```python
from build123d import *

# Parameters (mm, degrees)
SKETCH1_R           = 4.5
BOSS_EXTRUDE1_DEPTH = 5
SKETCH2_W           = 20
SKETCH2_H           = 39
BOSS_EXTRUDE2_DEPTH = 25
CUT_EXTRUDE1_DEPTH  = 30
SKETCH4_R           = 2.6
SKETCH4_R_2         = 3.2
CUT_EXTRUDE2_DEPTH  = 10
FILLET1_R           = 2
FILLET2_R           = 1


with BuildPart() as part:
    # Sketch1 → Boss-Extrude1 (new body)
    with BuildSketch(Plane.XY):
        Polygon((-10, 10), (-10, -10), (-10, -11), (10, -11), (10, -10), (10, 10), (10, 44), (-10, 44), align=None)
        with Locations((0, -0.5)):
            Circle(SKETCH1_R, mode=Mode.SUBTRACT)
    extrude(amount=BOSS_EXTRUDE1_DEPTH)

    # Sketch2 → Boss-Extrude2 (add)
    with BuildSketch(Plane(origin=(0, 0, 0), x_dir=(-1, 0, 0), z_dir=(0, 0, -1))):
        with Locations((0, 29.5)):
            Rectangle(SKETCH2_W, SKETCH2_H)
    extrude(amount=BOSS_EXTRUDE2_DEPTH)

    # Sketch3 → Cut-Extrude1 (cut)
    with BuildSketch(Plane(origin=(10, 0, 0), x_dir=(0, 0, -1), z_dir=(1, 0, 0))):
        Polygon((0, 15), (-5, 15), (-5, 49), (20, 49), (20, 15), align=None)
    extrude(amount=-CUT_EXTRUDE1_DEPTH, mode=Mode.SUBTRACT)

    # Sketch4 → Cut-Extrude2 (cut)
    with BuildSketch(Plane.XY.offset(-20)):
        with Locations((0, 40)):
            Circle(SKETCH4_R)
        with Locations((0, 25)):
            Circle(SKETCH4_R_2)
    extrude(amount=-CUT_EXTRUDE2_DEPTH, mode=Mode.SUBTRACT)

    # Fillet1
    fillet1_edges = [part.edges().sort_by_distance(p)[0] for p in [
        (0, 15, -20),
    ]]
    fillet(fillet1_edges, radius=FILLET1_R)

    # Fillet2
    fillet2_edges = [part.edges().sort_by_distance(p)[0] for p in [
        (0, 15, 5),
    ]]
    fillet(fillet2_edges, radius=FILLET2_R)


solid = part.part
```
Check sheet for the modelled part. Datum: model origin and axes. Units: mm. A direction names the side the tool comes from. Coordinates: 2 decimals unless noted, no trailing zeros. Order: outer loops, then holes, each group sorted by start corner. A loop starts at its lowest first (then second) coordinate and runs counter-clockwise, first axis right, second up. Notation, with made-up numbers: (46, 86.5) -> (89, 86.5) arc R19 ccw to (89, 102.5) -> close; hole circle Ø11 at (41, 70). An arc over 180 degrees is marked (long way). Write item = value, one per line. Start each with the question number.
1) Material ranges on L1, parallel to Y at x = 0, z = -23.4; L2, parallel to Y at x = 0, z = 1.5; L3, parallel to Y at x = -7.25, z = -14, recorded low to high.
2) Cross-section at A-A (y = -0.5). Enter the section's corners in (x, z).
3) Go/stop test with flat-tipped pins: P1, Ø3, axis at x = 3.5, z = -16.5, coming from the +Y side; P2, Ø10, axis at x = -2.5, y = -1.5, coming from the -Z side; P3, Ø6, axis at x = 1.5, z = -21, coming from the -Y side; P4, Ø8, axis at x = 0, y = -0.5, coming from the +Z side. Record where each tip stops, or that it passes through.
4) Mould release check, pull along X, two halves, no side actions. Record for faces 1 (the flat face through (-10, 14, -11)), 2 (the cylindrical face through (-0.417, 28.173, -22.465)), 3 (the flat face through (0, 33, -20)): +X half, -X half, draft (parallel to the pull), parting line (faces both ways), or undercut.
5) Cross-section at B-B (x = 0). Enter the section's corners in (y, z).
6) Access from +Z, -Z, +X, -X, +Y, -Y to the whole of each face (thin tool, end or side, straight path). Record for faces 4 (the flat face through (0, 15, -7)), 5 (the flat face through (-5, 0, 0)), 6 (the flat face through (10, 14, -11)).
7) Cross-section at C-C (z = -20.75). Enter the section's corners in (x, y), then the cut area to 3 significant figures.
8) Cross-section at D-D (y = 25). Enter the section's corners in (x, z).
Ans:
q1.L1 = 10 to 21.8, 28.2 to 37.4, 42.6 to 49
q1.L2 = -11 to -5, 4 to 15
q1.L3 = 10 to 15
q2.outline = (-10, 0) -> (-4.5, 0) -> (-4.5, 5) -> (-10, 5) -> close; (4.5, 0) -> (10, 0) -> (10, 5) -> (4.5, 5) -> close
q3.P1 = 15
q3.P2 = 0
q3.P3 = 10
q3.P4 = through
q4.face_1 = -X half
q4.face_2 = undercut
q4.face_3 = draft
q5.outline = (-11, 0) -> (-5, 0) -> (-5, 5) -> (-11, 5) -> close; (4, 0) -> (10, 0) -> (10, -25) -> (21.8, -25) -> (21.8, -20) -> (17, -20) arc R2 cw to (15, -18) -> (15, 4) arc R1 ccw to (14, 5) -> (4, 5) -> close; (28.2, -25) -> (37.4, -25) -> (37.4, -20) -> (28.2, -20) -> close; (42.6, -25) -> (49, -25) -> (49, -20) -> (42.6, -20) -> close
q6.face_4 = +Z, +X, -X, +Y
q6.face_5 = -Z, +X, -X, -Y
q6.face_6 = +Z, -Z, +X, +Y, -Y
q7.outline = (-10, 10) -> (10, 10) -> (10, 49) -> (-10, 49) -> close; hole circle Ø6.4 at (0, 25); hole circle Ø5.2 at (0, 40)
q7.area = 727 mm²
q8.outline = (-10, -25) -> (-3.2, -25) -> (-3.2, -20) -> (-10, -20) -> close; (3.2, -25) -> (10, -25) -> (10, -20) -> (3.2, -20) -> close
